Read the model definition and answer for the solid it produces. Units are mm, in the model's axes. Face numbers are marked on the shaded views. A direction names the side the tool comes from. Round coordinates to 2 decimals unless told otherwise and drop trailing zeros. Write each loop counter-clockwise with the first axis right and the second up, starting at its lowest first coordinate (ties: lowest second). Pieces come first, ordered by that corner, then holes. Notation, with made-up numbers: (3.5, -40) -> (59.5, -40) arc R21 ccw to (59.5, -21) -> close; hole circle Ø2 at (-5.75, -6.75). An arc over 180 degrees is marked (long way). Return JSON: item names as keys, results as strings. Group by question number.
(1) For the marked faces 4, 5, 6, 7 and 8, determine the directions among +Z, -Z, +X, -X, +Y, -Y from which every point of the face is accessible in a straight line to the end or side of a thin tool.
(2) Straight lines are drawn through the part: line 1 (X direction, y = -5, z = -18); line 2 (Y direction, x = 74.5, z = 0); line 3 (Y direction, x = 19, z = 0). For each, find the intervals that lie inside material, in ascending order.
(3) A cutting plane is placed at A-A on x = 76. Give the vertices of the cut face in (y, z), then the cut area to 3 significant figures.
(4) A cutting plane is placed at B-B on x = 19. Give the vertices of the cut face in (y, z).
(5) Given pin 1 (10 mm diameter, centred on x = 45, z = -13, fed in from +Y); pin 2 (15.5 mm diameter, centred on y = 0, z = 0, fed in from +X); pin 3 (1 mm diameter, centred on y = 11, z = -21.5, fed in from -X); pin 4 (1 mm diameter, centred on y = -24, z = 22, fed in from +X), each flat-ended and moving along its own axis, determine where each tip first touches the part or whether it passes through.
(6) The mould has two halves that part along Y. Classify the marked faces 1, 2 and 3: released by +Y, released by -Y, zero draft, split by the parting line, or undercut.
```python
from build123d import *

# Parameters (mm, degrees)
F4_R = 5.99999


# Not quite as in the source:
# - a fillet or chamfer is up to 0.001 mm smaller than in the source, because OpenCascade refuses the exact size


with BuildPart() as f1:
    # F0 (on Front) → F1 (revolve)
    with BuildSketch(Plane.XZ):
        with BuildLine():
            Line((0, 31), (0, 0))
            Line((0, 0), (88, 0))
            Line((88, 0), (88, 15))
            Line((88, 15), (85, 15))
            Line((85, 15), (85, 20))
            Line((85, 20), (68, 20))
            Line((68, 20), (68, 31))
            Line((68, 31), (56, 31))
            ThreePointArc((56, 31), (50, 25), (44, 31))
            Line((44, 31), (0, 31))
        make_face()
    revolve(axis=Axis((48.1394192929, 0, 0), (1, 0, 0)))

    # F2 (on Front) → F3 (revolve, cut)
    with BuildSketch(Plane.XZ):
        Polygon((0, 25), (0, 0), (88, 0), (88, 6), (30, 6), (30, 16), (22, 16), (22, 20.5), (15, 20.5), (15, 12.5), (12, 12.5), (12, 16), (1.5, 16), (1.5, 25), align=None)
    revolve(axis=Axis((-13.0126860076, 0, 0), (-1, 0, 0)), mode=Mode.SUBTRACT)

    # F4 (radius 6 in the source; OpenCascade refuses exactly that, so slightly less here)
    f4_edges = [f1.edges().sort_by_distance(p)[0] for p in [
        (0, 0, -31),
    ]]
    fillet(f4_edges, radius=F4_R)


solid = f1.part
```
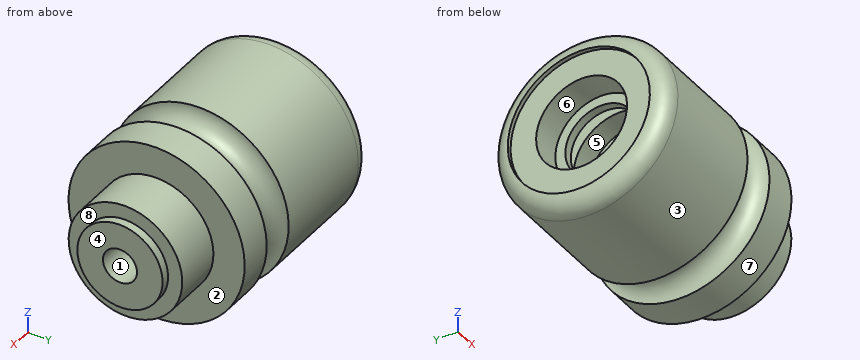
Checks:
{
 "1": {"face 4": "+Z, -Z, +X, +Y, -Y", "face 5": "none", "face 6": "-X", "face 7": "+X, -X", "face 8": "+X"},
 "2": {"line 1": "x = 1.5 to 15, 22 to 85", "line 2": "y = -20 to -6, 6 to 20", "line 3": "y = -31 to -20.5, 20.5 to 31"},
 "3": {"outline": "circle Ø40 at (0, 0); hole circle Ø12 at (0, 0)", "area": "1,140 mm^2"},
 "4": {"outline": "circle Ø62 at (0, 0); hole circle Ø41 at (0, 0)"},
 "5": {"pin 1": "stops at y = 29.92", "pin 2": "stops at x = 88", "pin 3": "stops at x = 1.5", "pin 4": "passes through"},
 "6": {"face 1": "undercut", "face 2": "zero draft", "face 3": "split by the parting line"}
}
